Check sheet for the modelled part. Datum: model origin and axes. Units: mm. A direction names the side the tool comes from. Give positions to 0.01 mm unless a question says otherwise; leave off trailing zeros. Order: outer loops, then holes, each group sorted by start corner. A loop starts at its lowest first (then second) coordinate and runs counter-clockwise, first axis right, second up.
```python
from build123d import *

# Parameters (mm, degrees)
SZKIC1_W                     = 60
SZKIC1_H                     = 60
DODANIE_WYCI_GNI_CIE1_DEPTH  = 100
SZKIC2_W                     = 57.5
SZKIC2_H                     = 57.5
WYTNIJ_WYCI_GNI_CIE1_DEPTH   = 6
SZKIC3_R                     = 5
WYTNIJ_WYCI_GNI_CIE2_DEPTH   = 24
SZKIC4_R                     = 19
WYTNIJ_WYCI_GNI_CIE3_DEPTH   = 0.9
ZAOKR_GLENIE1_R              = 1
OTWORY_USTALAJ_CE_6_0MM1_D   = 6
SZKIC8_R                     = 21
WYTNIJ_WYCI_GNI_CIE5_DEPTH   = 70
ZAOKR_GLENIE2_R              = 1
OTW_R_POD_RUB_M81_AT_2_COUNT = 2
OTW_R_POD_RUB_M81_AT_2_PITCH = 30
OTW_R_POD_RUB_M81_AT_3_COUNT = 2
OTW_R_POD_RUB_M81_AT_3_PITCH = 67.082039325
OTW_R_POD_RUB_M81_AT_4_COUNT = 2
OTW_R_POD_RUB_M81_AT_4_PITCH = 60


with BuildPart() as part:
    # Szkic1 → Dodanie-wyciągnięcie1 (new body)
    with BuildSketch(Plane(origin=(0, 0, 0), x_dir=(1, 0, 0), z_dir=(0, 1, 0))):
        Rectangle(SZKIC1_W, SZKIC1_H)
    extrude(amount=DODANIE_WYCI_GNI_CIE1_DEPTH)

    # Szkic2 → Wytnij-wyciągnięcie1 (cut)
    with BuildSketch(Plane(origin=(0, 100, 0), x_dir=(1, 0, 0), z_dir=(0, 1, 0))):
        Rectangle(SZKIC2_W, SZKIC2_H)
    extrude(amount=-WYTNIJ_WYCI_GNI_CIE1_DEPTH, mode=Mode.SUBTRACT)

    # Szkic3 → Wytnij-wyciągnięcie2 (cut)
    with BuildSketch(Plane(origin=(0, 94, 0), x_dir=(1, 0, 0), z_dir=(0, 1, 0))):
        with Locations(Location((0, 0, 0), (0, 0, 270))):
            Circle(SZKIC3_R)
    extrude(amount=-WYTNIJ_WYCI_GNI_CIE2_DEPTH, mode=Mode.SUBTRACT)

    # Szkic4 → Wytnij-wyciągnięcie3 (cut)
    with BuildSketch(Plane(origin=(0, 94, 0), x_dir=(1, 0, 0), z_dir=(0, 1, 0))):
        with Locations(Location((0, 0, 0), (0, 0, 270))):
            Circle(SZKIC4_R)
    extrude(amount=-WYTNIJ_WYCI_GNI_CIE3_DEPTH, mode=Mode.SUBTRACT)

    # Zaokrąglenie1
    # the kernel refuses this fillet: 1 mm, written as the material it adds along each edge
    with BuildSketch(Plane(origin=(0, 93.1, 0), x_dir=(0, 0, 1), z_dir=(-1, 0, 0))) as zaokr_glenie1_piece_1:
        with BuildLine():
            CenterArc((18.005012563, 1), ZAOKR_GLENIE1_R, 270, 84.260829523)
            Line((18.005012563, 0), (18.005012563, -0.02))
            Line((18.005012563, -0.02), (19, -0.02))
            Line((19, -0.02), (19.02, 0))
            ThreePointArc((19.02, 0), (19.02, 0.45), (19.019899749, 0.898))
            Line((19.019899749, 0.898), (19, 0.9))
        make_face()
    revolve(axis=Axis((0, 93.1, 0), (0, 1, 0)))

    # Otwory ustalające Ø6.0mm1 (through all)
    with Locations(Plane(origin=(0, 94, 0), x_dir=(1, 0, 0), z_dir=(0, 1, 0))):
        with Locations((-24, 24), (24, 24), (24, -24), (-24, -24)):
            Hole(OTWORY_USTALAJ_CE_6_0MM1_D / 2)

    # Szkic8 → Wytnij-wyciągnięcie5 (cut)
    with BuildSketch(Plane.XZ):
        with Locations(Location((0, 0, 0), (0, 0, 270))):
            Circle(SZKIC8_R)
    extrude(amount=-WYTNIJ_WYCI_GNI_CIE5_DEPTH, mode=Mode.SUBTRACT)

    # Zaokrąglenie2
    zaokr_glenie2_edges = [part.edges().sort_by_distance(p)[0] for p in [
        (30, 100, 0),
        (0, 100, -30),
        (-30, 100, 0),
        (0, 0, -30),
        (30, 0, 0),
        (0, 0, 30),
        (-30, 0, 0),
        (-30, 50, -30),
        (30, 50, -30),
        (30, 50, 30),
        (-30, 50, 30),
        (0, 100, 30),
    ]]
    fillet(zaokr_glenie2_edges, radius=ZAOKR_GLENIE2_R)

    # Szkic11 → Otwór pod śrubę M81 (revolve, cut)
    with BuildSketch(Plane(origin=(15, 80, -30), x_dir=(0, 1, 0), z_dir=(1, 0, 0))):
        Polygon((0, 0), (0, 12.703872786), (4.5, 10), (4.5, 0), align=None)
    otw_r_pod_rub_m81 = revolve(axis=Axis((15, 80, -36.35), (0, 0, 1)), mode=Mode.SUBTRACT)

    # Otwór pod śrubę M81 at 2: Otwór pod śrubę M81 ×2
    with Locations(*[(-i * OTW_R_POD_RUB_M81_AT_2_PITCH, 0, 0) for i in range(1, OTW_R_POD_RUB_M81_AT_2_COUNT)]):
        add(otw_r_pod_rub_m81, mode=Mode.SUBTRACT)

    # Otwór pod śrubę M81 at 3: Otwór pod śrubę M81 ×2
    with Locations(*[Vector(-0.4472135954999577, -0.894427190999916, 0) * (i * OTW_R_POD_RUB_M81_AT_3_PITCH) for i in range(1, OTW_R_POD_RUB_M81_AT_3_COUNT)]):
        add(otw_r_pod_rub_m81, mode=Mode.SUBTRACT)

    # Otwór pod śrubę M81 at 4: Otwór pod śrubę M81 ×2
    with Locations(*[(0, -i * OTW_R_POD_RUB_M81_AT_4_PITCH, 0) for i in range(1, OTW_R_POD_RUB_M81_AT_4_COUNT)]):
        add(otw_r_pod_rub_m81, mode=Mode.SUBTRACT)

    # Lustro1: Otwór pod śrubę M81 across plane
    add(otw_r_pod_rub_m81.mirror(Plane.XY), mode=Mode.SUBTRACT)

    # Lustro1 copy 1 sketch → Lustro1 copy 1 (revolve, cut)
    with BuildSketch(Plane(origin=(-15, 80, 30), x_dir=(0, 1, 0), z_dir=(1, 0, 0))):
        Polygon((0, 0), (0, -12.703872786), (4.5, -10), (4.5, 0), align=None)
    revolve(axis=Axis((-15, 80, 36.35), (0, 0, 1)), mode=Mode.SUBTRACT)

    # Lustro1 copy 2 sketch → Lustro1 copy 2 (revolve, cut)
    with BuildSketch(Plane(origin=(-15, 20, 30), x_dir=(0, 1, 0), z_dir=(1, 0, 0))):
        Polygon((0, 0), (0, -12.703872786), (4.5, -10), (4.5, 0), align=None)
    revolve(axis=Axis((-15, 20, 36.35), (0, 0, 1)), mode=Mode.SUBTRACT)

    # Lustro1 copy 3 sketch → Lustro1 copy 3 (revolve, cut)
    with BuildSketch(Plane(origin=(15, 20, 30), x_dir=(0, 1, 0), z_dir=(1, 0, 0))):
        Polygon((0, 0), (0, -12.703872786), (4.5, -10), (4.5, 0), align=None)
    revolve(axis=Axis((15, 20, 36.35), (0, 0, 1)), mode=Mode.SUBTRACT)


solid = part.part
```
(1) Cross-section at A-A on z = -24. Enter the section's corners in (x, y), then the cut area to 3 significant figures.
Response values:
outline: (-30, 1) arc R1 ccw to (-29, 0) - (-27, 0) - (-27, 94) - (-28.75, 94) - (-28.75, 100) - (-29, 100) arc R1 ccw to (-30, 99) - close; (-21, 0) - (21, 0) - (21, 94) - (-21, 94) - close; (27, 0) - (29, 0) arc R1 ccw to (30, 1) - (30, 99) arc R1 ccw to (29, 100) - (28.75, 100) - (28.75, 94) - (27, 94) - close; hole circle Ø9 at (-15, 20); hole circle Ø9 at (-15, 80); hole circle Ø9 at (15, 20); hole circle Ø9 at (15, 80)
area: 4,270 mm2
(2) Release check for a two-part mould opening along Z. For faces 1 (the face through (27, 46, -24)), 2 (the face through (30, 49, 0)), 3 (the face through (14.966, 79.219, -17.766)) record: released by +Z, released by -Z, zero draft, split by the parting line, or undercut.
Response values:
face 1: undercut
face 2: zero draft
face 3: released by -Z
(3) Cross-section at D-D on x = 24. Enter the section's corners in (y, z).
Response values:
outline: (0, -29) arc R1 ccw to (1, -30) - (99, -30) arc R1 ccw to (100, -29) - (100, -28.75) - (94, -28.75) - (94, -27) - (0, -27) - close; (0, -21) - (94, -21) - (94, 21) - (0, 21) - close; (0, 27) - (94, 27) - (94, 28.75) - (100, 28.75) - (100, 29) arc R1 ccw to (99, 30) - (1, 30) arc R1 ccw to (0, 29) - close
(4) Cross-section at C-C on y = 7. Enter the section's corners in (x, z).
Response values:
outline: (-30, -29) arc R1 ccw to (-29, -30) - (29, -30) arc R1 ccw to (30, -29) - (30, 29) arc R1 ccw to (29, 30) - (-29, 30) arc R1 ccw to (-30, 29) - close; hole circle Ø6 at (-24, -24); hole circle Ø6 at (-24, 24); hole circle Ø42 at (0, 0); hole circle Ø6 at (24, -24); hole circle Ø6 at (24, 24)
(5) Cross-section at B-B on z = 0. Enter the section's corners in (x, y), then the cut area to 3 significant figures.
Response values:
outline: (-30, 1) arc R1 ccw to (-29, 0) - (-21, 0) - (-21, 70) - (-5, 70) - (-5, 93.1) - (-18.01, 93.1) arc R1 cw to (-19, 94) - (-28.75, 94) - (-28.75, 100) - (-29, 100) arc R1 ccw to (-30, 99) - close; (5, 70) - (21, 70) - (21, 0) - (29, 0) arc R1 ccw to (30, 1) - (30, 99) arc R1 ccw to (29, 100) - (28.75, 100) - (28.75, 94) - (19, 94) arc R1 cw to (18.01, 93.1) - (5, 93.1) - close
area: 2,450 mm2
(6) Material ranges on L1, parallel to X at y = 20, z = -27.25; L2, parallel to Z at x = -24, y = 64; L3, parallel to Y at x = -15, z = 22.5, recorded low to high.
Response values:
L1: x = -30 to -19.5, -10.5 to 10.5, 19.5 to 30
L2: z = -30 to -27, -21 to 21, 27 to 30
L3: y = 0 to 15.5, 24.5 to 75.5, 84.5 to 94
(7) Set-up check for faces 4 (the face through (14.802, 75.504, 25.07)), 5 (the face through (28.75, 97, 0)), 6 (the face through (-15.198, 75.504, -25.07)), 7 (the face through (6.31, 34.51, -20.03)): record each of +Z, -Z, +X, -X, +Y, -Y from which the full face is reachable in a straight line by a thin tool's end or side.
Response values:
face 4: +Z
face 5: +Y
face 6: -Z
face 7: -Y
(8) Gauge pin test, flat ends, axial feed: pin 1 Ø8 at (x, z) = (24, 24) entering from +Y; pin 2 Ø7 at (x, y) = (-15, 80) entering from -Z; pin 3 Ø3 at (x, z) = (-4, -16) entering from -Y. Record the tip position at first contact, or that the pin passes through.
Response values:
pin 1: stops at y = 94
pin 2: stops at z = -19.4
pin 3: stops at y = 70
